```python
from build123d import *

# Parameters (mm, degrees)
F0_W     = 736.6
F0_H     = 38.1
F1_DEPTH = 76.2
F2_W     = 44.45
F2_H     = 19.05
F3_DEPTH = 152.401
F4_W     = 44.45
F4_H     = 38.1
F4_W_2   = 38.1
F5_DEPTH = 38.101
F6_W     = 38.1
F6_H     = 38.1
F7_DEPTH = 571.5


with BuildPart() as f1:
    # F0 (on Front) → F1 (new body, symmetric)
    with BuildSketch(Plane.XZ):
        Rectangle(F0_W, F0_H)
    extrude(amount=F1_DEPTH, both=True)

    # F2 (on face) → F3 (cut, through all)
    with BuildSketch(Plane.XZ.offset(76.2)):
        with Locations((-346.075, -9.525)):
            Rectangle(F2_W, F2_H)
        with Locations((346.075, -9.525)):
            Rectangle(F2_W, F2_H)
    extrude(amount=-F3_DEPTH, mode=Mode.SUBTRACT)

    # F4 (on face) → F5 (cut, through all)
    with BuildSketch(Plane(origin=(0, 0, -19.05), x_dir=(1, 0, 0), z_dir=(0, 0, -1))):
        with Locations((-346.075, 57.15)):
            Rectangle(F4_W, F4_H)
        with Locations((-304.8, 57.15)):
            Rectangle(F4_W_2, F4_H)
        with Locations((304.8, 57.15)):
            Rectangle(F4_W_2, F4_H)
        with Locations((346.075, 57.15)):
            Rectangle(F4_W, F4_H)
    extrude(amount=-F5_DEPTH, mode=Mode.SUBTRACT)

    # F6 (on face) → F7 (join, through all)
    with BuildSketch(Plane(origin=(-285.75, 0, 0), x_dir=(0, -1, 0), z_dir=(-1, 0, 0))):
        with Locations((57.15, -38.1)):
            Rectangle(F6_W, F6_H)
    extrude(amount=-F7_DEPTH)


solid = f1.part
```
Can you work these out from the model? Positions are in its coordinate system, mm. A direction names the side the tool comes from. Give positions to 0.01 mm unless a question says otherwise; leave off trailing zeros. Write each loop counter-clockwise with the first axis right and the second up, starting at its lowest first coordinate (ties: lowest second). Pieces come first, ordered by that corner, then holes. Notation, with made-up numbers: (16.25, -34) - (47.25, -34) arc R22 ccw to (47.25, -7) - close; hole circle Ø9 at (80, 19). An arc over 180 degrees is marked (long way). Write item = value, one per line. Start each with the question number.
1. Please list where these lines run through material, in increasing order: line 1 (Z direction, x = 202.5, y = -15.5); line 2 (X direction, y = 0.5, z = -16.5); line 3 (Y direction, x = 21, z = -37).
2. Imagine slicing it at A-A (z = 9.5). Please give me the cut outline in (x, y).
3. Imagine slicing it at D-D (z = -39). Please give me the cut outline in (x, y).
4. For pin 1 (6 mm diameter, centred on x = 150.5, y = 44, fed in from -Z); pin 2 (19 mm diameter, centred on x = 343.5, z = 4, fed in from -Y); pin 3 (11.5 mm diameter, centred on y = -53.5, z = -27.5, fed in from +X); pin 4 (15 mm diameter, centred on y = 0, z = -5.5, fed in from -X), each with a flat end and sliding along its axis, tell me the tip position at first contact or that it passes through.
5. Imagine slicing it at B-B (y = -30). Please give me the cut outline in (x, z).
6. On a 3-axis mill with a long thin cutter (end or side, diameter ignored), from which of +Z, -Z, +X, -X, +Y, -Y can I reach the whole of each face in a straight line? I mean faces 1 (the face through (-323.85, 18, -10)), 2 (the face through (285.75, -57, -19)), 3 (the face through (323.85, 18, -10)), 4 (the face through (-4, -38.1, -38)), 5 (the face through (-285.75, -57, -19)). Say none if no direction works.
7. Imagine slicing it at C-C (x = 276). Please give me the cut outline in (y, z), and give its area (3 significant figures).
Worked answers:
q1.line_1 = -19.05 to 19.05
q1.line_2 = -323.85 to 323.85
q1.line_3 = -76.2 to -38.1
q2.outline = (-368.3, -38.1) - (-285.75, -38.1) - (-285.75, -76.2) - (285.75, -76.2) - (285.75, -38.1) - (368.3, -38.1) - (368.3, 76.2) - (-368.3, 76.2) - close
q3.outline = (-285.75, -76.2) - (285.75, -76.2) - (285.75, -38.1) - (-285.75, -38.1) - close
q4.pin_1 = -19.05
q4.pin_2 = -38.1
q4.pin_3 = 285.75
q4.pin_4 = -368.3
q5.outline = (-368.3, 0) - (-323.85, 0) - (-323.85, -19.05) - (323.85, -19.05) - (323.85, 0) - (368.3, 0) - (368.3, 19.05) - (-368.3, 19.05) - close
q6.face_1 = -Z, -X, +Y, -Y
q6.face_2 = +Z, -Z, +X, -Y
q6.face_3 = -Z, +X, +Y, -Y
q6.face_4 = -Z, +X, -X, +Y
q6.face_5 = +Z, -Z, -X, -Y
q7.outline = (-76.2, -57.15) - (-38.1, -57.15) - (-38.1, -19.05) - (76.2, -19.05) - (76.2, 19.05) - (-76.2, 19.05) - close
q7.area = 7,260 mm2
